For this review, take the finished solid that the model builds, in its own axes (mm). Face numbers are marked on the shaded views. A direction names the side the tool comes from. Give positions to 0.01 mm unless a question says otherwise; leave off trailing zeros. Write each loop counter-clockwise with the first axis right and the second up, starting at its lowest first coordinate (ties: lowest second). Pieces come first, ordered by that corner, then holes.
1) Machinability: for the marked faces 1 and 2, which of the approach directions +Z, -Z, +X, -X, +Y, -Y give a long, thin tool a straight path to every point of the face, cutting with its end or side? Answer none if there is none.
2) We need section D-D on x = 17.5. Give the boundary of the cut face in (y, z), and give its area (3 significant figures).
3) We need section B-B on x = 33.5. Give the boundary of the cut face in (y, z).
4) Wall thickness on line 1 along Y through (x, z) = (3.5, 8); line 2 along X through (y, z) = (32.5, 24); line 3 along Z through (x, y) = (34, 32.5): over which ranges is each line inside the solid? List them lowest first.
5) We need section C-C on z = 37.5. Give the boundary of the cut face in (x, y), and give its area (3 significant figures).
6) For P1, Ø22, axis at y = 33.5, z = 22.5, coming from the -X side; P2, Ø22, axis at x = 6, z = 24.5, coming from the +Y side, all flat-tipped, find the tip position at first contact; note any pin that passes through.
7) We need section A-A on z = 31.5. Give the boundary of the cut face in (x, y).
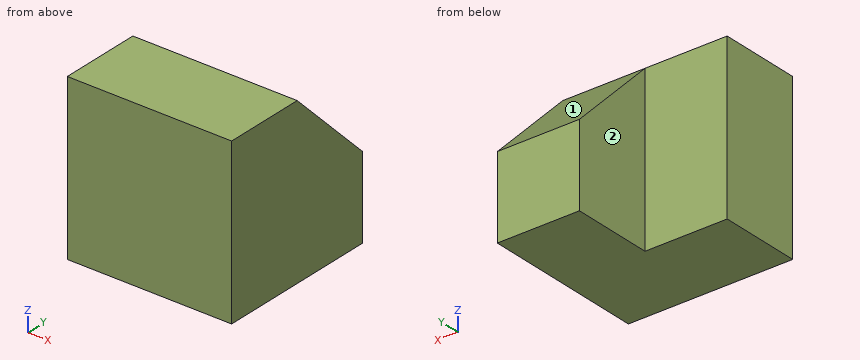
from build123d import *

# Parameters (mm, degrees)
SKETCH1_W           = 40
SKETCH1_H           = 40
BOSS_EXTRUDE1_DEPTH = 40
SKETCH2_W           = 20
SKETCH2_H           = 20
CUT_EXTRUDE1_DEPTH  = 40
CUT_EXTRUDE2_DEPTH  = 40


with BuildPart() as part:
    # Sketch1 → Boss-Extrude1 (new body)
    with BuildSketch(Plane.XY):
        with Locations((20, 20)):
            Rectangle(SKETCH1_W, SKETCH1_H)
    extrude(amount=BOSS_EXTRUDE1_DEPTH)

    # Sketch2 → Cut-Extrude1 (cut)
    with BuildSketch(Plane.XY.offset(40)):
        with Locations((10, 30)):
            Rectangle(SKETCH2_W, SKETCH2_H)
    extrude(amount=-CUT_EXTRUDE1_DEPTH, mode=Mode.SUBTRACT)

    # Sketch3 → Cut-Extrude2 (cut)
    with BuildSketch(Plane.ZY.offset(-20)):
        Polygon((20, 40), (40, 20), (40, 40), align=None)
    extrude(amount=-CUT_EXTRUDE2_DEPTH, mode=Mode.SUBTRACT)


solid = part.part
Results list:
1. face 1: +Z, +X, -X, +Y
1. face 2: +Z, -Z, -X, +Y
2. outline: (0, 0) - (20, 0) - (20, 40) - (0, 40) - close
2. area: 800 mm2
3. outline: (0, 0) - (40, 0) - (40, 20) - (20, 40) - (0, 40) - close
4. line 1: y = 0 to 20
4. line 2: x = 20 to 40
4. line 3: z = 0 to 27.5
5. outline: (0, 0) - (40, 0) - (40, 22.5) - (20, 22.5) - (20, 20) - (0, 20) - close
5. area: 850 mm2
6. P1: stops at x = 20
6. P2: stops at y = 20
7. outline: (0, 0) - (40, 0) - (40, 28.5) - (20, 28.5) - (20, 20) - (0, 20) - close
